from build123d import *

# Parameters (mm, degrees)
F0_W     = 119.956396
F0_H     = 118.582852
F0_R     = 25.815734
F1_DEPTH = 10
F2_R     = 20


with BuildPart() as f1:
    # F0 (on Front) → F1 (new body)
    with BuildSketch(Plane.XZ):
        Rectangle(F0_W, F0_H)
        with Locations((0, -1.831395)):
            Circle(F0_R, mode=Mode.SUBTRACT)
    extrude(amount=F1_DEPTH)

    # F2
    f2_edges = [f1.edges().sort_by_distance(p)[0] for p in [
        (-59.978198, -5, 59.291426),
        (59.978198, -5, 59.291426),
        (-59.978198, -5, -59.291426),
        (59.978198, -5, -59.291426),
    ]]
    fillet(f2_edges, radius=F2_R)


solid = f1.part
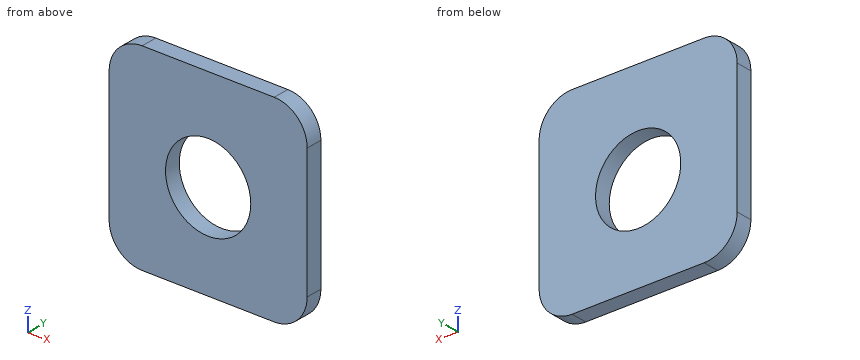
Here's how the part is built. I have some questions about the finished solid (model axes, mm). Round coordinates to 2 decimals unless told otherwise and drop trailing zeros. Write each loop counter-clockwise with the first axis right and the second up, starting at its lowest first coordinate (ties: lowest second). Pieces come first, ordered by that corner, then holes. Notation, with made-up numbers: (56.5, 1) -> (73.5, 1) arc R34 cw to (73.5, 38) -> close; hole circle Ø3 at (79.5, -15). An arc over 180 degrees is marked (long way). One line per item, written item: value.
1) Suppose I cut it at B-B on z = -10.5. List the corners of the cut face in (x, y) for me.
Filled sheet:
outline: (-59.98, -10) -> (-24.32, -10) -> (-24.32, 0) -> (-59.98, 0) -> close; (24.32, -10) -> (59.98, -10) -> (59.98, 0) -> (24.32, 0) -> close
2) Suppose I cut it at C-C on y = -4.5. List the corners of the cut face in (x, z) for me.
Filled sheet:
outline: (-59.98, -39.29) arc R20 ccw to (-39.98, -59.29) -> (39.98, -59.29) arc R20 ccw to (59.98, -39.29) -> (59.98, 39.29) arc R20 ccw to (39.98, 59.29) -> (-39.98, 59.29) arc R20 ccw to (-59.98, 39.29) -> close; hole circle Ø51.63 at (0, -1.83)
3) If I drill on line 1 (Z direction, x = 0, y = -4.25); line 2 (X direction, y = -4.75, z = -2.5); line 3 (X direction, y = -1, z = -11), over which ranges is the centre line in solid material (lowest first)? Write a range as [from, to].
Filled sheet:
line 1: z = [-59.29, -27.65], [23.98, 59.29]
line 2: x = [-59.98, -25.81], [25.81, 59.98]
line 3: x = [-59.98, -24.13], [24.13, 59.98]
4) Suppose I cut it at D-D on z = -51. List the corners of the cut face in (x, y) for me.
Filled sheet:
outline: (-56.19, -10) -> (56.19, -10) -> (56.19, 0) -> (-56.19, 0) -> close
5) Suppose I cut it at A-A on x = 0. List the corners of the cut face in (y, z) for me.
Filled sheet:
outline: (-10, -59.29) -> (0, -59.29) -> (0, -27.65) -> (-10, -27.65) -> close; (-10, 23.98) -> (0, 23.98) -> (0, 59.29) -> (-10, 59.29) -> close
6) I'm going to push a flat-ended pin straight in: pin 1 Ø5 at (y, z) = (-7.5, 45.5) entering from -X. Where does the tip first touch, or does it pass through?
Filled sheet:
pin 1: stops at x = -59.63
